Part model, mm, in its own coordinate system. Face numbers are marked on the shaded views. Give positions to 0.01 mm unless a question says otherwise; leave off trailing zeros. Write each loop counter-clockwise with the first axis right and the second up, starting at its lowest first coordinate (ties: lowest second). Pieces come first, ordered by that corner, then holes. Notation, with made-up numbers: M -26.75,-26.5 L 26.25,-26.5 A20 cw 26.25,12.5 Z; hole C 66,78 d8. An arc over 180 degrees is marked long. Use CSV: the item, a comma, the result in double quotes. Start each with the question number.
Item 1: Pin check, flat tip, straight feed: pin 1 (4.5 mm diameter, centred on x = 0, z = -15, fed in from -Y). Stop position of the tip, or through.
Item 2: Cut at C-C (z = 0). List the corners of the cut face in (x, y), then the cut area to 3 significant figures.
Item 3: Cut at B-B (y = 8.5). List the corners of the cut face in (x, z).
Item 4: Mould opens along Z. For the marked faces 1, 2, 3 and 4 say: released by +Z, released by -Z, zero draft, split by the parting line, or undercut.
Item 5: Cut at D-D (x = 0). List the corners of the cut face in (y, z).
Item 6: Cut at A-A (z = -15). List the corners of the cut face in (x, y).
Item 7: Drill centre lines: line 1 (Z direction, x = 0, y = 6.25); line 2 (Z direction, x = 2.5, y = 5); line 3 (Y direction, x = -6.65, z = 0). Where is each one in solid material? Low to high. Write a range as [from, to].
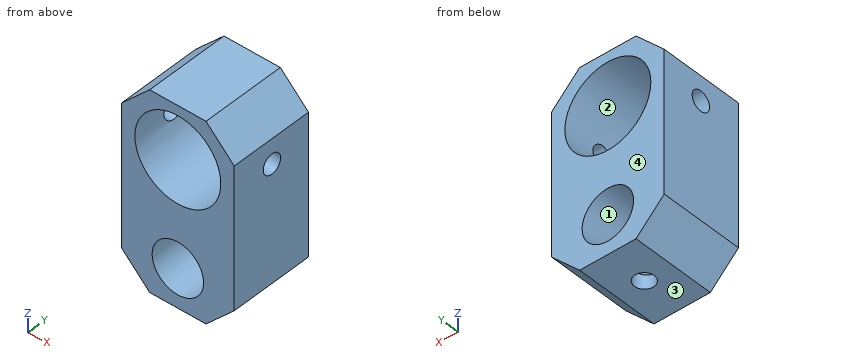
Autodesk Inventor part; units mm, degrees
ref_plane "YZ Plane" through (0, 0, 0) normal (1, 0, 0) x (0, 1, 0)
ref_plane "XZ Plane" through (0, 0, 0) normal (0, 1, 0) x (-1, 0, 0)
ref_plane "XY Plane" through (0, 0, 0) normal (0, 0, 1) x (1, 0, 0)
sketch "Sketch1" plane through (0, 0, 0) normal (0, 1, 0) x (-1, 0, 0)
  circle A0 centre (0, 0) radius 6.1
  circle A1 centre (0, -15) radius 3.65
  line L0 (8, 7.5) -> (-8, 7.5)
  line L1 (-8, 7.5) -> (-8, -20.5)
  line L2 (-8, -20.5) -> (8, -20.5)
  line L3 (8, -20.5) -> (8, 7.5)
  dimension "d0" = 12.2
  dimension "d1" = 7.3
  dimension "d2" = 15
  dimension "d3" = 16
  dimension "d4" = 8
  dimension "d5" = 28
  dimension "d6" = 5.5
extrude "Extrusion1" add sketch "Sketch1" along normal blind 12
chamfer "Chamfer1" distance 4 angle 45 4 edges at (8, 6, -20.5) (-8, 6, -20.5) (8, 6, 7.5) (-8, 6, 7.5)
sketch "Sketch3" plane through (8, 0, 3.5) normal (1, 0, 0) x (0, 0, -1)
  line L0 (-4, 12) -> (-4, 0)
  point P0 (3.5, 0)
  point P1 (3.5, 6.0888)
  dimension "d12" = 7.5
hole "Hole1" at (8, 6.0888, 0) direction (-1, 0, 0) diameter 2.8 depth 17.75
sketch "Sketch4" plane through (4, 0, -20.5) normal (0, 0, -1) x (-1, 0, 0)
  line L0 (8, 12) -> (8, 0)
  line L1 (0, 0) -> (8, 0)
  point P0 (4, 0)
  point P1 (4, 6.1062)
  dimension "d20" = 4
  dimension "d21" = 6.1062
hole "Hole2" at (0, 6.1062, -20.5) direction (0, 0, 1) diameter 2.8 depth 5
properties part number "Z axis collar"
Worked answers:
1,pin 1,"passes through"
2,outline,"M -8,0 L -6.1,0 L -6.1,4.69 L -8,4.69 Z; M -8,7.49 L -6.1,7.49 L -6.1,12 L -8,12 Z; M 6.1,0 L 8,0 L 8,4.69 L 6.1,4.69 Z; M 6.1,7.49 L 8,7.49 L 8,12 L 6.1,12 Z"
2,area,"35.0 mm^2"
3,outline,"M -8,-16.5 L -4,-20.5 L 4,-20.5 L 8,-16.5 L 8,3.5 L 4,7.5 L -4,7.5 L -8,3.5 Z; hole C 0,0 d12.2; hole C 0,-15 d7.3"
4,face 1,"undercut"
4,face 2,"undercut"
4,face 3,"released by -Z"
4,face 4,"zero draft"
5,outline,"M 0,-20.5 L 4.71,-20.5 L 4.71,-18.65 L 0,-18.65 Z; M 0,-11.35 L 12,-11.35 L 12,-6.1 L 0,-6.1 Z; M 0,6.1 L 12,6.1 L 12,7.5 L 0,7.5 Z; M 7.51,-20.5 L 12,-20.5 L 12,-18.65 L 7.51,-18.65 Z"
6,outline,"M -8,0 L -3.65,0 L -3.65,12 L -8,12 Z; M 3.65,0 L 8,0 L 8,12 L 3.65,12 Z"
7,line 1,"z = [-11.35, -6.1], [6.1, 7.5]"
7,line 2,"z = [-20.5, -17.66], [-12.34, -5.56], [5.56, 7.5]"
7,line 3,"y = [0, 4.69], [7.49, 12]"
